Geometry: see drawing. Coordinates: mm, zero at the bounding-box minimum. Coordinates: 2 decimals unless noted, no trailing zeros. Loops run counter-clockwise (first coordinate to the right, second up) from the corner with the lowest first, then second, coordinate; pieces in that order, holes last. Notation, with made-up numbers: M 0.5,-19.5 L 34.5,-19.5 A18 ccw 34.5,-8.5 Z; hole C 61,33.5 d4. An arc over 180 degrees is marked long. One line per question, with ' | ' between items. Start each with the question number.
1. Pin query (flat end, axial travel): P1, Ø4, axis at y = 20.5, z = 5.5, coming from the -X side; P2, Ø1, axis at y = 4, z = 29.5, coming from the -X side; P3, Ø2, axis at x = 42.5, z = 32.5, coming from the -Y side. Return the tip coordinate at first contact, or that it passes through.
2. Section query C-C, the plane z = 3. Output: boundary loops of the cut face in (x, y), and give its area (3 significant figures).
3. Section query B-B, the plane x = 14. Output: boundary loops of the cut face in (y, z).
4. Ray query, probe 1 along X at (y, z) = (13.5, 29.5); probe 2 along Z at (x, y) = (19, 6.5) (3 decimals); probe 3 along X at (y, z) = (11, 36.5). Return the intervals inside material, ascending.
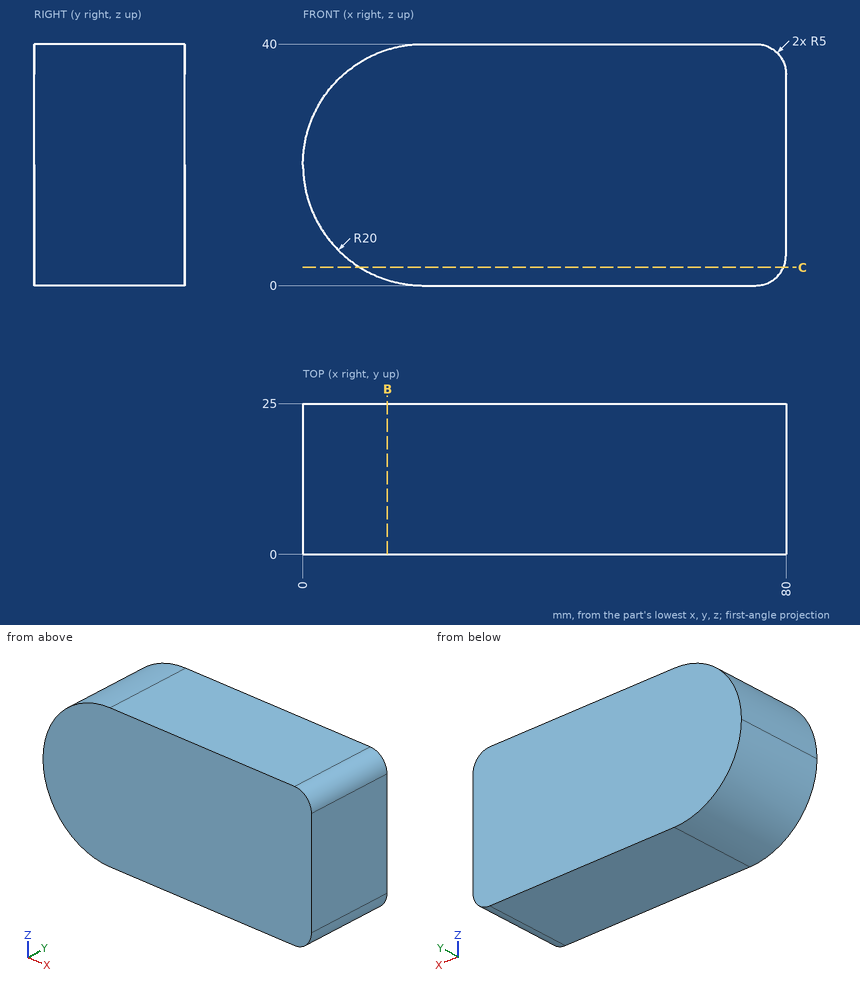
Taken from the geometry:
1) P1: x = 4.39 | P2: x = 2.14 | P3: y = 0
2) outline: M 9.46,0 L 79.58,0 L 79.58,25 L 9.46,25 Z | area: 1,750 mm^2
3) outline: M 0,0.92 L 25,0.92 L 25,39.08 L 0,39.08 Z
4) probe 1: 2.4 to 80 | probe 2: 0.025 to 39.975 | probe 3: 8.7 to 79.77
